The model under review builds one solid part; all positions refer to its coordinate system, in mm. Coordinates: 2 decimals unless noted, no trailing zeros. Loops run counter-clockwise (first coordinate to the right, second up) from the corner with the lowest first, then second, coordinate; pieces in that order, holes last. Notation, with made-up numbers: (69, 44.25) - (106, 44.25) arc R20 ccw to (106, 83.25) - close; hole circle Ø6 at (-31.75, 21). An arc over 180 degrees is marked (long way). Use a Markdown table: item, result. Add a question column.
1) Add section B-B, the plane y = 22.75. Give the boundary of the cut face in (x, z).
2) Clearance check with flat-ended pins moving along their axes: pin 1 (2 mm diameter, centred on y = 17, z = -1.5, fed in from +X); pin 2 (0.6 mm diameter, centred on y = 22.5, z = -2.5, fed in from +X). State where each tip first meets the part, or that it passes through.
3) The part is to be moulded in two halves that separate along Z. For faces 1 (the flat face through (0, 7, -3)), 2 (the cylindrical face through (0.751, 12.325, 2.385)), 3 (the flat face through (0, 25, 0)), say which applies: pulls with the +Z half, pulls with the -Z half, needs draft (parallel to the pull), parting line crosses it, or undercut.
4) Add section D-D, the plane y = 13.5. Give the boundary of the cut face in (x, z), and give its area (3 significant figures).
5) Add section C-C, the plane z = 1.85. Give the boundary of the cut face in (x, y).
6) To check wall thickness, follow L1, parallel to Z at x = -0.15, y = 9; L2, parallel to Z at x = -0.1, y = 2.75; L3, parallel to X at y = 4.5, z = 0.4. State the ranges of each line that lie inside material, in increasing order. Write a range as [from, to].
7) Add section A-A, the plane x = 0. Give the boundary of the cut face in (y, z).
```python
from build123d import *

# Parameters (mm, degrees)
SKETCH_1_R      = 2.5
EXTRUDE_1_DEPTH = 25
SKETCH_2_W      = 2
SKETCH_2_H      = 1
EXTRUDE_2_DEPTH = 8
EXTRUDE_START   = -5
EXTRUDE_3_DEPTH = 5


with BuildPart() as part:
    # 草图1 → 凸台-拉伸1 (new body)
    with BuildSketch(Plane(origin=(0, 0, 0), x_dir=(1, 0, 0), z_dir=(0, 1, 0))):
        with Locations(Location((0, 0, 0), (0, 0, 270))):
            Circle(SKETCH_1_R)
    extrude(amount=EXTRUDE_1_DEPTH)

    # 草图2 → 凸台-拉伸2 (add)
    with BuildSketch(Plane(origin=(0, 3, 0), x_dir=(-1, 0, 0), z_dir=(0, -1, 0))):
        with Locations((0, 2.5)):
            Rectangle(SKETCH_2_W, SKETCH_2_H)
    extrude(amount=-EXTRUDE_2_DEPTH)

    # 草图3 → 凸台-拉伸3 (add)
    with BuildSketch(Plane(origin=(0, 25, 0), x_dir=(1, 0, 0), z_dir=(0, 1, 0)).offset(EXTRUDE_START)):
        with BuildLine():
            Line((-1, 3), (-1, 2.291287847))
            ThreePointArc((-1, 2.291287847), (0, 2.5), (1, 2.291287847))
            Line((1, 2.291287847), (1, 3))
            Line((1, 3), (-1, 3))
        make_face()
    extrude(amount=EXTRUDE_3_DEPTH)


solid = part.part
```
From the geometry:
| question | item | result |
|---|---|---|
| 1 | outline | (-1, -3) - (1, -3) - (1, -2.29) arc R2.5 ccw (long way) to (-1, -2.29) - close |
| 2 | pin 1 | stops at x = 2.45 |
| 2 | pin 2 | stops at x = 1.19 |
| 3 | face 1 | pulls with the -Z half |
| 3 | face 2 | parting line crosses it |
| 3 | face 3 | needs draft |
| 4 | outline | circle Ø5 at (0, 0) |
| 4 | area | 19.6 mm^2 |
| 5 | outline | (-1.68, 0) - (1.68, 0) - (1.68, 25) - (-1.68, 25) - close |
| 6 | L1 | z = [-3, 2.5] |
| 6 | L2 | z = [-2.5, 2.5] |
| 6 | L3 | x = [-2.47, 2.47] |
| 7 | outline | (0, -2.5) - (3, -2.5) - (3, -3) - (11, -3) - (11, -2.5) - (20, -2.5) - (20, -3) - (25, -3) - (25, 2.5) - (0, 2.5) - close |
